from build123d import *

# Parameters (mm, degrees)
SKETCH1_R           = 50.8
SKETCH1_R_2         = 3.175
BOSS_EXTRUDE1_DEPTH = 38.1
CUT_EXTRUDE1_DEPTH  = 39.1


with BuildPart() as part:
    # Sketch1 → Boss-Extrude1 (new body)
    with BuildSketch(Plane(origin=(0, 0, 0), x_dir=(1, 0, 0), z_dir=(0, 1, 0))):
        Circle(SKETCH1_R)
        Circle(SKETCH1_R_2, mode=Mode.SUBTRACT)
    extrude(amount=BOSS_EXTRUDE1_DEPTH)

    # Sketch2 → Cut-Extrude1 (cut, through all)
    with BuildSketch(Plane(origin=(0, 38.1, 0), x_dir=(1, 0, 0), z_dir=(0, 1, 0))):
        with BuildLine():
            Line((-3.175, 3.174), (-3.175, 7.620000001))
            ThreePointArc((-3.175, 7.620000001), (0, 10.795), (3.175, 7.62))
            Line((3.175, 7.62), (3.175, 3.176))
            Line((3.175, 3.176), (7.621, 3.176))
            ThreePointArc((7.621, 3.176), (10.796, 0.001), (7.621, -3.174))
            Line((7.621, -3.174), (3.177, -3.174))
            Line((3.177, -3.174), (3.177, -7.62))
            ThreePointArc((3.177, -7.62), (0.002, -10.795), (-3.173, -7.62))
            Line((-3.173, -7.62), (-3.173, -3.176))
            Line((-3.173, -3.176), (-7.619, -3.176))
            ThreePointArc((-7.619, -3.176), (-10.794, -0.001), (-7.619, 3.174))
            Line((-7.619, 3.174), (-3.175, 3.174))
        make_face()
    extrude(amount=-CUT_EXTRUDE1_DEPTH, mode=Mode.SUBTRACT)


solid = part.part
For this review, take the finished solid that the model builds, in its own axes (mm). A direction names the side the tool comes from. Give positions to 0.01 mm unless a question says otherwise; leave off trailing zeros. Loops run counter-clockwise (first coordinate to the right, second up) from the corner with the lowest first, then second, coordinate; pieces in that order, holes last. Notation, with made-up numbers: M 61,-11 L 90,-11 A25 ccw 90,8 Z; hole C 14.5,23 d4. An arc over 180 degrees is marked long. Put each result on its own line as item: value. Start each with the question number.
(1) Add section A-A, the plane z = 0. Write out the cut boundary in (x, y).
(2) The part is to be moulded in two halves that separate along Z. For faces 1 (the flat face through (-1, 0, -12)), 2 (the cylindrical face through (-11.012, 18.783, 49.592)), 3 (the flat face through (5, 19, 3.174)), say which applies: +Z half, -Z half, draft (parallel to the pull), parting line (faces both ways), or undercut.
(3) For pin 1 (1.3 mm diameter, centred on x = -6.5, y = 27, fed in from +Z); pin 2 (5 mm diameter, centred on y = 18, z = -7.5, fed in from -X); pin 3 (3.5 mm diameter, centred on y = 11.5, z = -6.5, fed in from +X), all flat-tipped, find the tip position at first contact; note any pin that passes through.
(4) Wall thickness on L1, parallel to Z at x = 1.5, y = 25.5; L2, parallel to Z at x = -9, y = 9.5; L3, parallel to X at y = 35, z = -8.5: over which ranges is each line inside the solid? List them lowest first.
(5) Add section D-D, the plane x = 34. Write out the cut boundary in (y, z), then the cut area to 3 significant figures.
(6) Machinability: for faces 4 (the flat face through (-1, 38.1, -12)), 5 (the flat face through (-5, 19, 3.176)), which of the approach directions +Z, -Z, +X, -X, +Y, -Y give a long, thin tool a straight path to every point of the face, cutting with its end or side? Answer none if there is none.
(7) Add section C-C, the plane y = 34.5. Write out the cut boundary in (x, z) (3 decimals).
(8) Add section B-B, the plane x = 0. Write out the cut boundary in (y, z) (3 decimals).
Result:
1. outline: M -50.8,0 L -10.79,0 L -10.79,38.1 L -50.8,38.1 Z; M 10.8,0 L 50.8,0 L 50.8,38.1 L 10.8,38.1 Z
2. face 1: draft
2. face 2: parting line
2. face 3: undercut
3. pin 1: stops at z = 50.46
3. pin 2: stops at x = -50.55
3. pin 3: stops at x = 50.58
4. L1: z = -50.78 to -10.42, 10.42 to 50.78
4. L2: z = -50 to -2.86, 2.86 to 50
4. L3: x = -50.08 to -3.05, 3.05 to 50.08
5. outline: M 0,-37.74 L 38.1,-37.74 L 38.1,37.74 L 0,37.74 Z
5. area: 2,880 mm^2
6. face 4: +Z, -Z, +X, -X, +Y
6. face 5: +Y, -Y
7. outline: C 0,0 d101.6; hole M -7.619,-3.174 L -3.175,-3.174 L -3.175,-7.62 A3.175 ccw 3.175,-7.62 L 3.175,-3.176 L 7.621,-3.176 A3.175 ccw 7.621,3.174 L 3.177,3.174 L 3.177,7.62 A3.175 ccw -3.173,7.62 L -3.173,3.176 L -7.619,3.176 A3.175 ccw Z
8. outline: M 0,-50.8 L 38.1,-50.8 L 38.1,-10.795 L 0,-10.795 Z; M 0,10.795 L 38.1,10.795 L 38.1,50.8 L 0,50.8 Z
